Could you check a few things on this model? Use its own coordinates, in mm. A direction names the side the tool comes from. Give positions to 0.01 mm unless a question says otherwise; leave off trailing zeros. Order: outer loops, then holes, each group sorted by start corner. A loop starts at its lowest first (then second) coordinate and runs counter-clockwise, first axis right, second up. Notation, with made-up numbers: (45, 27) - (60, 27) arc R10 cw to (60, 41) - close; hole circle Ø3 at (27, 19.5). An arc over 180 degrees is marked (long way). One line per question, with ' | ' between items. Start each with the question number.
1. I need wall thicknesses on probe 1 along X at (y, z) = (18.5, 17); probe 2 along Z at (x, y) = (-38, 5); probe 3 along Z at (x, y) = (-37, 11). Which ranges of each line are inside material? Lowest first, please. Write a range as from..to.
2. Imagine slicing it at A-A (x = -42.5). Please give me the cut outline in (y, z), and give its area (3 significant figures).
3. Imagine slicing it at B-B (z = -60). Please give me the cut outline in (x, y).
4. Which directions (+Z, -Z, +X, -X, +Y, -Y) give clear straight access to the entire face, cutting with the end or side of a thin tool? Please do faces 4 (the flat face through (-28, 32.7, 66)), 5 (the cylindrical face through (45.649, 18.585, -82.042)), 6 (the flat face through (44, 11.7, 27)), 7 (the flat face through (54, 14, -18)), 8 (the flat face through (-56, 15, 56)).
5. If we mould it in two halves opening along X, with no side actions, what happens to faces 1 (the flat face through (-33, 13, 53)), 2 (the flat face through (57.5, 14, -21)), 3 (the flat face through (-35, 3, -13.357))? For each: released by +X, released by -X, zero draft, split by the parting line, or undercut.
6. Imagine slicing it at C-C (x = 1). Please give me the cut outline in (y, z), and give its area (3 significant figures).
7. Imagine slicing it at D-D (z = 65). Please give me the cut outline in (x, y), and give its area (3 significant figures).
8. For P1, Ø5, axis at x = 42.5, z = 25, coming from the +Y side; P2, Ø9, axis at x = -13, y = 27, coming from the +Z side; P3, Ø1.8, axis at x = -56, y = 16.5, coming from the +Z side, each with a flat end and sliding along its axis, tell me the tip position at first contact or that it passes through.
```python
from build123d import *

# Parameters (mm, degrees)
SKETCH1_W                               = 115
SKETCH1_H                               = 170
BACK_WALL_EXTRUDE_DEPTH                 = 6
SKETCH2_W                               = 115
SKETCH2_H                               = 6
BOTTOM_PLATE_EXTRUDE_DEPTH              = 30
SKETCH3_W                               = 3.5
SKETCH3_H                               = 135
SIDE_WALLS_EXTRUDE_DEPTH                = 20
SKETCH4_W                               = 16.3
SKETCH4_H                               = 23.5
DIAL_INDIACTOR_HOLDER_EXTRUDE_DEPTH     = 26.7
SKETCH6_R                               = 3
DIAL_INDICATOR_TIGHTENER_HOLE_CUT_DEPTH = 26.7
DIAL_INDICATOR_HOLDER_CUT_DEPTH         = 30
SKETCH7_R                               = 5.1
ARM_BASE_EXTRUDE_DEPTH                  = 5.7
SKETCH8_R                               = 3
ARM_AXLE_EXTRUDE_DEPTH                  = 7.6
SKETCH9_R                               = 5.1
GUIDE_WHEEL_BASE_EXTRUDE_DEPTH          = 3.5
SKETCH10_R                              = 2.45
GUIDE_WHEEL_AXLE_EXTRUDE_DEPTH          = 8
FILAMENT_SLOT_CUT_DEPTH                 = 116
SKETCH13_R                              = 3.96875
MOUNTING_HOLES_CUT_DEPTH                = 8
FILLET1_R                               = 2
SKETCH15_R                              = 1.3
SCREW_HOLE_CUT_DEPTH                    = 20.3
WEIGHT_REDUCTION_CUT_REACH              = 8
WEIGHT_REDUCTION_CUT_2_DEPTH            = 20


with BuildPart() as part:
    # Sketch1 → Back Wall Extrude (new body)
    with BuildSketch(Plane(origin=(0, 0, 0), x_dir=(1, 0, 0), z_dir=(0, 1, 0))):
        Rectangle(SKETCH1_W, SKETCH1_H)
    extrude(amount=BACK_WALL_EXTRUDE_DEPTH)

    # Sketch2 → Bottom Plate Extrude (add)
    with BuildSketch(Plane(origin=(0, 6, 0), x_dir=(1, 0, 0), z_dir=(0, 1, 0))):
        with Locations((0, 82)):
            Rectangle(SKETCH2_W, SKETCH2_H)
    extrude(amount=BOTTOM_PLATE_EXTRUDE_DEPTH)

    # Sketch3 → Side Walls Extrude (add)
    with BuildSketch(Plane(origin=(0, 6, 0), x_dir=(1, 0, 0), z_dir=(0, 1, 0))):
        with Locations((-55.75, 11.5)):
            Rectangle(SKETCH3_W, SKETCH3_H)
        with Locations((55.75, 11.5)):
            Rectangle(SKETCH3_W, SKETCH3_H)
    extrude(amount=SIDE_WALLS_EXTRUDE_DEPTH)

    # Sketch4 → Dial Indiactor Holder Extrude (add)
    with BuildSketch(Plane(origin=(0, 6, 0), x_dir=(1, 0, 0), z_dir=(0, 1, 0))):
        with Locations((-32.65, -64.75)):
            Rectangle(SKETCH4_W, SKETCH4_H)
    extrude(amount=DIAL_INDIACTOR_HOLDER_EXTRUDE_DEPTH)

    # Sketch6 → Dial Indicator Tightener Hole Cut (cut)
    with BuildSketch(Plane.ZY.offset(40.8)):
        with Locations((64.75, 26.7)):
            Circle(SKETCH6_R)
    extrude(amount=-DIAL_INDICATOR_TIGHTENER_HOLE_CUT_DEPTH, mode=Mode.SUBTRACT)

    # Sketch18 → Dial Indicator Holder Cut (cut)
    with BuildSketch(Plane.XY.offset(76.5)):
        with BuildLine():
            Line((-33.9, 32.7), (-31.4, 32.7))
            Line((-31.4, 32.7), (-31.4, 22.765337686))
            ThreePointArc((-31.4, 22.765337686), (-32.775371215, 13.450428626), (-33.9, 22.798925129))
            Line((-33.9, 22.798925129), (-33.9, 32.7))
        make_face()
    extrude(amount=-DIAL_INDICATOR_HOLDER_CUT_DEPTH, mode=Mode.SUBTRACT)

    # Sketch7 → Arm Base Extrude (add)
    with BuildSketch(Plane(origin=(0, 6, 0), x_dir=(1, 0, 0), z_dir=(0, 1, 0))):
        with Locations((41.6, -24.9)):
            Circle(SKETCH7_R)
    extrude(amount=ARM_BASE_EXTRUDE_DEPTH)

    # Sketch8 → Arm Axle Extrude (add)
    with BuildSketch(Plane(origin=(0, 11.7, 0), x_dir=(1, 0, 0), z_dir=(0, 1, 0))):
        with Locations((41.6, -24.9)):
            Circle(SKETCH8_R)
    extrude(amount=ARM_AXLE_EXTRUDE_DEPTH)

    # Sketch9 → Guide Wheel Base Extrude (add)
    with BuildSketch(Plane(origin=(0, 6, 0), x_dir=(1, 0, 0), z_dir=(0, 1, 0))):
        with Locations((-32.6, 4.4)):
            Circle(SKETCH9_R)
    extrude(amount=GUIDE_WHEEL_BASE_EXTRUDE_DEPTH)

    # Sketch10 → Guide Wheel Axle Extrude (add)
    with BuildSketch(Plane(origin=(0, 9.5, 0), x_dir=(1, 0, 0), z_dir=(0, 1, 0))):
        with Locations((-32.6, 4.4)):
            Circle(SKETCH10_R)
    extrude(amount=GUIDE_WHEEL_AXLE_EXTRUDE_DEPTH)

    # Sketch11 → Filament Slot Cut (cut, through all)
    with BuildSketch(Plane.ZY.offset(57.5)):
        with BuildLine():
            Line((14, 12.765586), (7, 12.765586))
            ThreePointArc((7, 12.765586), (4.5, 15.265586), (7, 17.765586))
            Line((7, 17.765586), (14, 17.765586))
            ThreePointArc((14, 17.765586), (16.5, 15.265586), (14, 12.765586))
        make_face()
    extrude(amount=-FILAMENT_SLOT_CUT_DEPTH, mode=Mode.SUBTRACT)

    # Sketch13 → Mounting Holes Cut (cut)
    with BuildSketch(Plane(origin=(0, 0, -85), x_dir=(-1, 0, 0), z_dir=(0, 0, -1))):
        with Locations((42.5, 21)):
            Circle(SKETCH13_R)
        with Locations((-42.5, 21)):
            Circle(SKETCH13_R)
    extrude(amount=-MOUNTING_HOLES_CUT_DEPTH, mode=Mode.SUBTRACT)

    # Fillet1
    fillet1_edges = [part.edges().sort_by_distance(p)[0] for p in [
        (-55.75, 26, 56),
        (-55.75, 26, -79),
        (55.75, 26, -79),
        (55.75, 26, 56),
        (-27.95, 32.7, 53),
        (-37.35, 32.7, 53),
        (-57.5, 3, 85),
    ]]
    fillet(fillet1_edges, radius=FILLET1_R)

    # Sketch15 → Screw Hole Cut (cut, through all)
    with BuildSketch(Plane(origin=(0, 19.3, 0), x_dir=(1, 0, 0), z_dir=(0, 1, 0))):
        with Locations((41.6, -24.9)):
            Circle(SKETCH15_R)
    extrude(amount=-SCREW_HOLE_CUT_DEPTH, mode=Mode.SUBTRACT)

    # Sketch21 → Weight Reduction Cut (cut, up to next)
    with BuildSketch(Plane(origin=(0, 6, 0), x_dir=(1, 0, 0), z_dir=(0, 1, 0)), mode=Mode.PRIVATE) as weight_reduction_cut_sk1:
        Polygon((-48.44610903, 73.348314607), (48.898876404, 73.348314607), (48.898876404, 13.356637536), (48.898876404, -8.639749456), (27.392426134, -8.639749456), (27.392426134, -40.975447357), (-21.053682896, -63.034891603), (-21.053682896, 13.356637536), (-48.44610903, 13.356637536), align=None)
    weight_reduction_cut_tool1 = extrude(weight_reduction_cut_sk1.sketch, amount=-WEIGHT_REDUCTION_CUT_REACH, mode=Mode.PRIVATE) & part.part
    add(weight_reduction_cut_tool1.solids().sort_by_distance((2.646642, 6, -20.266546))[0], mode=Mode.SUBTRACT)

    # Sketch22 → Weight Reduction Cut 2 (cut, symmetric)
    with BuildSketch(Plane(origin=(0, 6, 0), x_dir=(1, 0, 0), z_dir=(0, 1, 0))):
        Polygon((57.5, -40.74906367), (-24.5, -76.5), (-57.5, -76.5), (-57.5, -85), (57.5, -85), align=None)
    extrude(amount=WEIGHT_REDUCTION_CUT_2_DEPTH, both=True, mode=Mode.SUBTRACT)


solid = part.part
```
Results found:
1) probe 1: x = -57.5..-54, 54..57.5 | probe 2: z = -85..-73.35, -13.36..76.5 | probe 3: z = -85..-79, 53..76.5
2) outline: (0, -85) - (17.03, -85) - (17.03, -79) - (6, -79) - (6, -73.35) - (0, -73.35) - close; (0, -13.36) - (6, -13.36) - (6, 76.5) - (0, 76.5) - close; (24.97, -85) - (36, -85) - (36, -79) - (24.97, -79) - close | area: 741 mm2
3) outline: (-57.5, 0) - (-48.45, 0) - (-48.45, 6) - (-54, 6) - (-54, 26) - (-57.5, 26) - close; (48.9, 0) - (57.5, 0) - (57.5, 26) - (54, 26) - (54, 6) - (48.9, 6) - close
4) face 4: +Z, +X, -X, +Y | face 5: -Z | face 6: +Y | face 7: +Z, +Y | face 8: +Z, -X, +Y
5) face 1: zero draft | face 2: released by +X | face 3: undercut
6) outline: (0, -85) - (36, -85) - (36, -79) - (6, -79) - (6, -73.35) - (0, -73.35) - close; (0, 52.99) - (6, 52.99) - (6, 65.38) - (0, 65.38) - close | area: 324 mm2
7) outline: (-57.5, 0) - (1.88, 0) - (1.88, 6) - (-24.5, 6) - (-24.5, 23.71) - (-31.4, 23.71) - (-31.4, 22.77) arc R4.75 cw (long way) to (-33.9, 22.8) - (-33.9, 23.71) - (-40.8, 23.71) - (-40.8, 6) - (-57.5, 6) - close; (-40.8, 29.69) - (-33.9, 29.69) - (-33.9, 32.7) - (-40.8, 32.7) - close; (-31.4, 29.69) - (-24.5, 29.69) - (-24.5, 32.7) - (-31.4, 32.7) - close | area: 614 mm2
8) P1: stops at y = 19.3 | P2: stops at z = -79 | P3: stops at z = 56
